Read the model definition and answer for the solid it produces. Units are mm, in the model's axes. A direction names the side the tool comes from. Round coordinates to 2 decimals unless told otherwise and drop trailing zeros. Loops run counter-clockwise (first coordinate to the right, second up) from the corner with the lowest first, then second, coordinate; pieces in that order, holes last. Notation, with made-up numbers: M 16.25,-40 L 28.25,-40 A25 cw 28.25,-19 Z; hole C 85,-7.75 d5. An arc over 180 degrees is marked long. Write each question's results on one line, items separated by ' | '.
Autodesk Inventor part; units mm, degrees
ref_plane "YZ Plane" through (0, 0, 0) normal (1, 0, 0) x (0, 1, 0)
ref_plane "XZ Plane" through (0, 0, 0) normal (0, 1, 0) x (-1, 0, 0)
ref_plane "XY Plane" through (0, 0, 0) normal (0, 0, 1) x (1, 0, 0)
sketch "Sketch1" plane through (0, 0, 0) normal (0, 1, 0) x (-1, 0, 0)
  circle A0 centre (0, 0) radius 7.9375
  dimension "d0" = 15.875
extrude "Extrusion1" add sketch "Sketch1" along normal blind 76.2
sketch "Sketch2" plane through (0, 76.2, 0) normal (0, 1, 0) x (1, 0, 0)
  circle A0 centre (0, 0) radius 4.5
  dimension "d3" = 9
extrude "Extrusion2" cut sketch "Sketch2" against normal blind 3
chamfer "Chamfer1" distance 3 angle 45 1 edges at (-4.5, 76.2, 0)
sketch "Sketch3" plane through (0, 0, 0) normal (0, -1, 0) x (1, 0, 0)
  circle A0 centre (0, 2) radius 1.5
  circle A1 centre (0, -2) radius 1.5
  point P0 (0, 0)
  dimension "d9" = 3
  dimension "d10" = 3
  dimension "d11" = 2
  dimension "d12" = 2
extrude "Extrusion3" add sketch "Sketch3" along normal blind 15
properties part number "Heater630W" material "Steel, Alloy"
Item 1: The part is cut by section B-B (y = -3). Determine the outline of the cut face in (x, z).
Outcome:
outline: C 0,-2 d3; C 0,2 d3
Item 2: The mould has two halves that part along Z. Classify faces 1 (the face through (-0.195, -7.395, 0.513)), 2 (the face through (0, -15, -2)), 3 (the face through (1.72, 37.57, 7.75)): pulls with the +Z half, pulls with the -Z half, needs draft (parallel to the pull), parting line crosses it, or undercut.
Outcome:
face 1: undercut | face 2: needs draft | face 3: parting line crosses it
Item 3: Flat-ended cylindrical pins translate along their axes: pin 1 (5 mm diameter, centred on y = 59, z = 3, fed in from +X); pin 2 (2 mm diameter, centred on x = 3.5, y = 4.5, fed in from -Z); pin 3 (4 mm diameter, centred on y = 12, z = -6, fed in from +X). Find the tip coordinate at first contact, or state that the pin passes through.
Outcome:
pin 1: stops at x = 7.92 | pin 2: stops at z = -7.53 | pin 3: stops at x = 6.86
Item 4: Straight lines are drawn through the part: line 1 (Y direction, x = -0.5, z = 2.25); line 2 (Y direction, x = -2.75, z = -7); line 3 (X direction, y = 25.5, z = -0.25). For each, find the intervals that lie inside material, in ascending order.
Outcome:
line 1: y = -15 to 73.2 | line 2: y = 0 to 76.2 | line 3: x = -7.93 to 7.93
Item 5: The part is cut by section C-C (y = 54). Determine the outline of the cut face in (x, z) (1 decimal), plus the area to 3 significant figures.
Outcome:
outline: C 0,0 d15.9 | area: 198 mm2
Item 6: For faces 4 (the face through (0, -15, 2)), 5 (the face through (-0.325, -7.395, -0.536)), 6 (the face through (0, 73.2, 0)), determine the directions among +Z, -Z, +X, -X, +Y, -Y from which every point of the face is accessible in a straight line to the end or side of a thin tool.
Outcome:
face 4: +Z, -Z, +X, -X, -Y | face 5: -Y | face 6: +Y
